Read the model definition and answer for the solid it produces. Units are mm, in the model's axes. A direction names the side the tool comes from. Coordinates: 2 decimals unless noted, no trailing zeros. Write each loop counter-clockwise with the first axis right and the second up, starting at its lowest first coordinate (ties: lowest second). Pieces come first, ordered by that corner, then holes. Notation, with made-up numbers: (30.5, 62) - (74.5, 62) arc R15 ccw to (74.5, 82) - close; hole circle Ø4 at (-6.75, 52). An arc over 180 degrees is marked (long way). Use a Markdown table: item, result.
from build123d import *

# Parameters (mm, degrees)
F0_W     = 300
F0_H     = 100
F1_DEPTH = 9
F2_W     = 12
F2_H     = 12
F3_DEPTH = 300.001
F4_R     = 5.99999
F5_R     = 1.49999


# Not quite as in the source:
# - a fillet or chamfer is up to 0.001 mm smaller than in the source, because OpenCascade refuses the exact size


with BuildPart() as f1:
    # F0 (on Front) → F1 (new body, symmetric)
    with BuildSketch(Plane.XZ):
        with Locations((-3.7248600274, -105.7776198197)):
            Rectangle(F0_W, F0_H)
    extrude(amount=F1_DEPTH, both=True)

    # F2 (on face) → F3 (cut, through all)
    with BuildSketch(Plane.YZ.offset(146.2751399726)):
        with Locations((0, -61.7776198197)):
            Rectangle(F2_W, F2_H)
    extrude(amount=-F3_DEPTH, mode=Mode.SUBTRACT)

    # F4 (radius 6 in the source; OpenCascade refuses exactly that, so slightly less here)
    f4_edges = [f1.edges().sort_by_distance(p)[0] for p in [
        (-3.72486, 6, -67.77762),
        (-3.72486, -6, -67.77762),
    ]]
    fillet(f4_edges, radius=F4_R)

    # F5 (radius 1.5 in the source; OpenCascade refuses exactly that, so slightly less here)
    f5_edges = [f1.edges().sort_by_distance(p)[0] for p in [
        (-3.72486, -9, -55.77762),
        (-3.72486, -6, -55.77762),
        (-3.72486, 6, -55.77762),
        (-3.72486, 9, -55.77762),
    ]]
    fillet(f5_edges, radius=F5_R)


solid = f1.part
(1) This flat-tipped pin is pushed along its axis until it touches: P1, Ø10, axis at x = 86.5, y = -6.5, coming from the +Z side. Where does it stop, or does it pass through?
Report:
| item | result |
|---|---|
| P1 | stops at z = -55.78 |
(2) A cutting plane is placed at B-B, the plane y = -3. Write down the section's boundary in (x, z).
Report:
| item | result |
|---|---|
| outline | (-153.72, -155.78) - (146.28, -155.78) - (146.28, -66.97) - (-153.72, -66.97) - close |
(3) Straight lines are drawn through the part: L1, parallel to Z at x = -71.5, y = 4.25; L2, parallel to Z at x = 64.5, y = 4.75. For each, find the intervals that lie inside material, in ascending order.
Report:
| item | result |
|---|---|
| L1 | z = -155.78 to -66.01 |
| L2 | z = -155.78 to -65.44 |
(4) The mould has two halves that part along Y. Classify faces 1 (the cylindrical face through (-5.82, -4.29, -65.97)), 2 (the flat face through (-6, -9, -106)), 3 (the flat face through (-6, 0, -155.778)): pulls with the +Y half, pulls with the -Y half, needs draft (parallel to the pull), parting line crosses it, or undercut.
Report:
| item | result |
|---|---|
| face 1 | undercut |
| face 2 | pulls with the -Y half |
| face 3 | needs draft |
(5) For faces 4 (the cylindrical face through (-5.825, 4.196, -66.067)), 5 (the flat face through (-153.725, 0, -106)), determine the directions among +Z, -Z, +X, -X, +Y, -Y from which every point of the face is accessible in a straight line to the end or side of a thin tool.
Report:
| item | result |
|---|---|
| face 4 | +Z, +X, -X |
| face 5 | +Z, -Z, -X, +Y, -Y |
